Can you work these out from the drawing? Everything is in mm from the part's minimum corner. A direction names the side the tool comes from. Round coordinates to 2 decimals unless told otherwise and drop trailing zeros. Loops run counter-clockwise (first coordinate to the right, second up) from the corner with the lowest first, then second, coordinate; pieces in that order, holes last. Notation, with made-up numbers: (12.25, -20.75) -> (55.25, -20.75) arc R8 ccw to (55.25, -11.75) -> close; hole circle Ø7 at (-27.5, 28). An arc over 180 degrees is marked (long way). Answer as a JSON object with one key per item and string values.
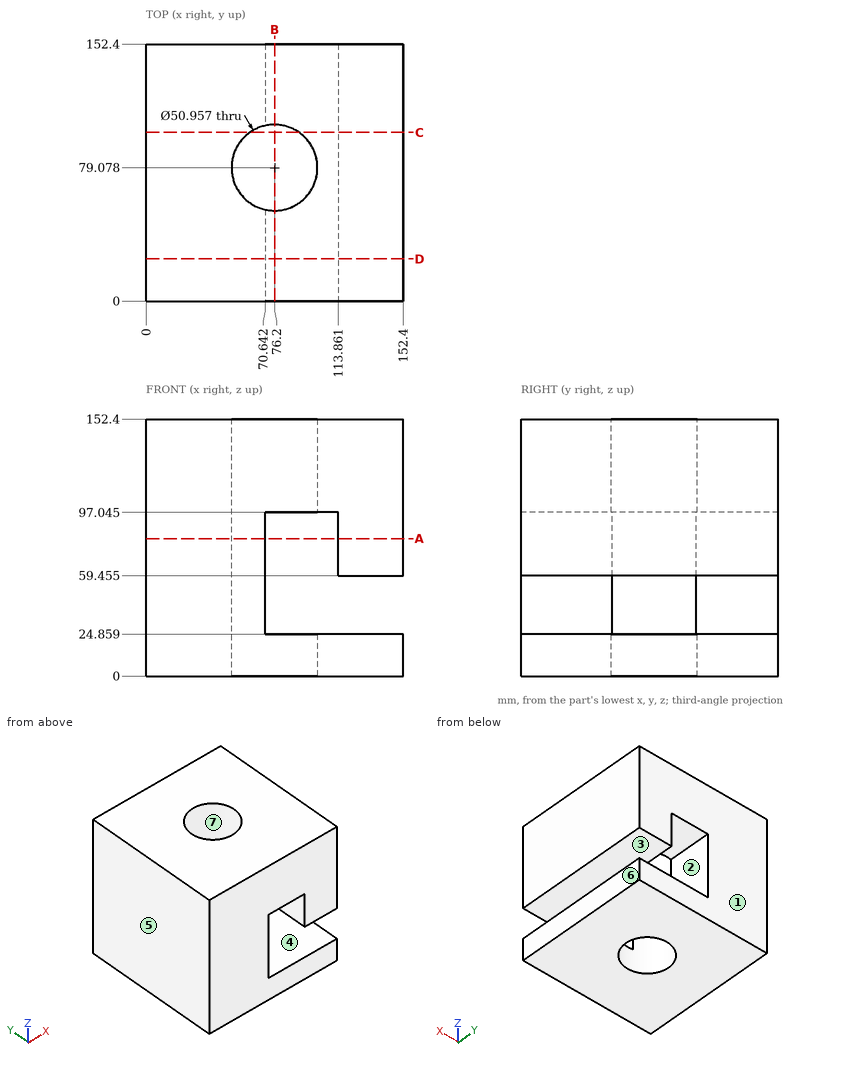
Q1. I want a section at C-C, the plane y = 100. Write out the boundary of the cut face in (x, z) (1 decimal).
Determined:
{"outline": "(0, 0) -> (61.7, 0) -> (61.7, 152.4) -> (0, 152.4) -> close; (90.7, 0) -> (152.4, 0) -> (152.4, 24.9) -> (90.7, 24.9) -> close; (90.7, 97) -> (113.9, 97) -> (113.9, 59.5) -> (152.4, 59.5) -> (152.4, 152.4) -> (90.7, 152.4) -> close"}
Q2. I want a section at D-D, the plane y = 25. Write out the boundary of the cut face in (x, z) (1 decimal).
Determined:
{"outline": "(0, 0) -> (152.4, 0) -> (152.4, 24.9) -> (70.6, 24.9) -> (70.6, 97) -> (113.9, 97) -> (113.9, 59.5) -> (152.4, 59.5) -> (152.4, 152.4) -> (0, 152.4) -> close"}
Q3. I want a section at B-B, the plane x = 76.2. Write out the boundary of the cut face in (y, z) (1 decimal), then the cut area to 3 significant figures.
Determined:
{"outline": "(0, 0) -> (53.6, 0) -> (53.6, 24.9) -> (0, 24.9) -> close; (0, 97) -> (53.6, 97) -> (53.6, 152.4) -> (0, 152.4) -> close; (104.6, 0) -> (152.4, 0) -> (152.4, 24.9) -> (104.6, 24.9) -> close; (104.6, 97) -> (152.4, 97) -> (152.4, 152.4) -> (104.6, 152.4) -> close", "area": "8,140 mm²"}
Q4. If I drill on L1, parallel to X at y = 25.5, z = 77; L2, parallel to Z at x = 108, y = 38 (1 decimal); L3, parallel to Z at x = 121, y = 134 (1 decimal), over which ranges is the centre line in solid material (lowest first)? Write a range as [from, to].
Determined:
{"L1": "[0, 70.64], [113.86, 152.4]", "L2": "[0, 24.9], [97, 152.4]", "L3": "[0, 24.9], [59.5, 152.4]"}
Q5. We'd pull the mould along X, two halves only. Please class the marked faces 4, 5, 6 and 7: pulls with the +X half, pulls with the -X half, needs draft (parallel to the pull), parting line crosses it, or undercut.
Determined:
{"face 4": "needs draft", "face 5": "pulls with the -X half", "face 6": "pulls with the +X half", "face 7": "undercut"}
Q6. I want a section at A-A, the plane z = 81.5. Write out the boundary of the cut face in (x, y).
Determined:
{"outline": "(0, 0) -> (70.64, 0) -> (70.64, 54.21) arc R25.48 cw to (70.64, 103.94) -> (70.64, 152.4) -> (0, 152.4) -> close; (113.86, 0) -> (152.4, 0) -> (152.4, 152.4) -> (113.86, 152.4) -> close"}
Q7. On a 3-axis mill with a long thin cutter (end or side, diameter ignored), from which of +Z, -Z, +X, -X, +Y, -Y can I reach the whole of each face in a straight line? I mean the marked faces 1, 2 and 3. Say none if no direction works.
Determined:
{"face 1": "+Z, -Z, +X, -X, +Y", "face 2": "+Y, -Y", "face 3": "+X, +Y, -Y"}
